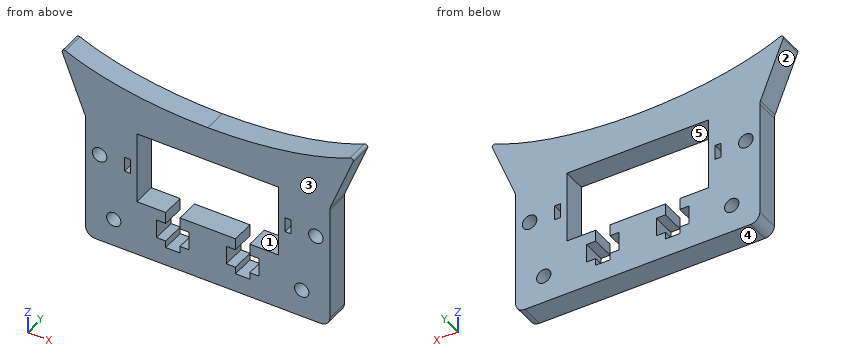
from build123d import *

# Parameters (mm, degrees)
SKETCH1_W           = 105
SKETCH1_H           = 70
BOSS_EXTRUDE1_DEPTH = 10
SKETCH2_W           = 61
SKETCH2_H           = 31
CUT_EXTRUDE1_DEPTH  = 11
SKETCH3_W           = 6.15
SKETCH3_H           = 5
SKETCH3_H_2         = 3
CUT_EXTRUDE2_DEPTH  = 10
SKETCH4_R           = 3.125
SKETCH4_W           = 2.5
SKETCH4_H           = 6.35
CUT_EXTRUDE3_DEPTH  = 11
BOSS_EXTRUDE2_DEPTH = 10
SKETCH6_R           = 3.075
CUT_EXTRUDE4_DEPTH  = 11.0000001
FILLET2_R           = 1
FILLET1_R           = 4


with BuildPart() as part:
    # Sketch1 → Boss-Extrude1 (new body)
    with BuildSketch(Plane(origin=(0, 0, 0), x_dir=(1, 0, 0), z_dir=(0, 1, 0))):
        Rectangle(SKETCH1_W, SKETCH1_H)
    extrude(amount=BOSS_EXTRUDE1_DEPTH)

    # Sketch2 → Cut-Extrude1 (cut, through all)
    with BuildSketch(Plane(origin=(0, 10, 0), x_dir=(1, 0, 0), z_dir=(0, 1, 0))):
        with Locations((0, -4.5)):
            Rectangle(SKETCH2_W, SKETCH2_H)
    extrude(amount=-CUT_EXTRUDE1_DEPTH, mode=Mode.SUBTRACT)

    # Sketch3 → Cut-Extrude2 (cut)
    with BuildSketch(Plane(origin=(0, 10, 0), x_dir=(1, 0, 0), z_dir=(0, 1, 0))):
        with Locations((-15, 13.5)):
            Rectangle(SKETCH3_W, SKETCH3_H)
        Polygon((-18.075, 24), (-22, 24), (-22, 16), (-18.075, 16), (-11.925, 16), (-8, 16), (-8, 24), (-11.925, 24), (-11.925, 21), (-18.075, 21), align=None)
        with Locations((-15, 22.5)):
            Rectangle(SKETCH3_W, SKETCH3_H_2)
        with Locations((-15, 25.5)):
            Rectangle(SKETCH3_W, SKETCH3_H_2)
    cut_extrude2 = extrude(amount=-CUT_EXTRUDE2_DEPTH, mode=Mode.SUBTRACT)

    # Sketch4 → Cut-Extrude3 (cut, through all)
    with BuildSketch(Plane(origin=(0, 10, 0), x_dir=(1, 0, 0), z_dir=(0, 1, 0))):
        with Locations((-46.5, -4)):
            Circle(SKETCH4_R)
        with Locations((-34.5, -4)):
            Rectangle(SKETCH4_W, SKETCH4_H)
    cut_extrude3 = extrude(amount=-CUT_EXTRUDE3_DEPTH, mode=Mode.SUBTRACT)

    # Sketch5 → Boss-Extrude2 (add)
    with BuildSketch(Plane(origin=(0, 0, 0), x_dir=(1, 0, 0), z_dir=(0, 1, 0))):
        with BuildLine():
            Line((0, -35), (-52.5, -19.039128985))
            Line((-52.5, -19.039128985), (-63.478993436, -46.742400328))
            add(Edge.make_bspline(
                [(0, -35), (-39.462588608, -35), (-63.478993436, -46.742400328)],
                knots=[4.71238898, 4.71238898, 4.71238898, 5.628907116, 5.628907116, 5.628907116], degree=2, weights=[1, 0.896824023, 1]))
        make_face()
    boss_extrude2 = extrude(amount=BOSS_EXTRUDE2_DEPTH)

    # Sketch6 → Cut-Extrude4 (cut, through all)
    with BuildSketch(Plane(origin=(0, 10, 0), x_dir=(1, 0, 0), z_dir=(0, 1, 0))):
        with Locations((-40.420875644, 23.095045258)):
            Circle(SKETCH6_R)
    cut_extrude4 = extrude(amount=-CUT_EXTRUDE4_DEPTH, mode=Mode.SUBTRACT)

    # Mirror1: Cut-Extrude2, Cut-Extrude3, Boss-Extrude2, Cut-Extrude4 across plane
    add(cut_extrude2.mirror(Plane(origin=(0, 0, 0), x_dir=(0, 0, 1), z_dir=(1, 0, 0))), mode=Mode.SUBTRACT)
    add(cut_extrude3.mirror(Plane(origin=(0, 0, 0), x_dir=(0, 0, 1), z_dir=(1, 0, 0))), mode=Mode.SUBTRACT)
    add(boss_extrude2.mirror(Plane(origin=(0, 0, 0), x_dir=(0, 0, 1), z_dir=(1, 0, 0))))
    add(cut_extrude4.mirror(Plane(origin=(0, 0, 0), x_dir=(0, 0, 1), z_dir=(1, 0, 0))), mode=Mode.SUBTRACT)

    # Fillet2
    fillet2_edges = [part.edges().sort_by_distance(p)[0] for p in [
        (-63.478993436, 5, 46.742400328),
        (63.478993436, 5, 46.742400328),
    ]]
    fillet(fillet2_edges, radius=FILLET2_R)

    # Fillet1
    fillet1_edges = [part.edges().sort_by_distance(p)[0] for p in [
        (52.5, 5, 19.039128985),
        (-52.5, 5, -35),
        (52.5, 5, -35),
        (-52.5, 5, 19.039128985),
    ]]
    fillet(fillet1_edges, radius=FILLET1_R)


solid = part.part
The listing builds one solid part. Answer for the finished solid, in the listing's coordinates (mm). Face numbers are marked on the shaded views. A direction names the side the tool comes from. Give positions to 0.01 mm unless a question says otherwise; leave off trailing zeros. Loops run counter-clockwise (first coordinate to the right, second up) from the corner with the lowest first, then second, coordinate; pieces in that order, holes last. Notation, with made-up numbers: M 13,68 L 46,68 A17 cw 46,93 Z; hole C -29,-26 d10. An arc over 180 degrees is marked long. Answer as CSV lines item,"result".
Item 1: The part is cut by section A-A (z = 4). Give the vertices of the cut face in (x, y) (3 decimals), and give its area (3 significant figures).
Values follow:
outline,"M -52.5,0 L -49.625,0 L -49.625,10 L -52.5,10 Z; M -43.375,0 L -35.75,0 L -35.75,10 L -43.375,10 Z; M -33.25,0 L -30.5,0 L -30.5,10 L -33.25,10 Z; M 30.5,0 L 33.25,0 L 33.25,10 L 30.5,10 Z; M 35.75,0 L 43.375,0 L 43.375,10 L 35.75,10 Z; M 49.625,0 L 52.5,0 L 52.5,10 L 49.625,10 Z"
area,"265 mm^2"
Item 2: Given pin 1 Ø3 at (y, z) = (7, -7.5) entering from -X; pin 2 Ø2 at (x, y) = (20.5, 4) entering from +Z; pin 3 Ø10 at (x, z) = (40.42, -23.1) entering from +Y; pin 4 Ø5 at (y, z) = (5.5, 31) entering from +X, each flat-ended and moving along its own axis, determine where each tip first touches the part or whether it passes through.
Values follow:
pin 1,"stops at x = -52.5"
pin 2,"stops at z = 36.1"
pin 3,"stops at y = 10"
pin 4,"stops at x = 58.23"
Item 3: Straight lines are drawn through the part: line 1 along X through (y, z) = (6.5, 4) (3 decimals); line 2 along Z through (x, y) = (-18, 3.25); line 3 along X through (y, z) = (8.75, -7). For each, find the intervals that lie inside material, in ascending order. Write a range as [from, to].
Values follow:
line 1,"x = [-52.5, -49.625], [-43.375, -35.75], [-33.25, -30.5], [30.5, 33.25], [35.75, 43.375], [49.625, 52.5]"
line 2,"z = [-35, -27], [20, 35.77]"
line 3,"x = [-52.5, -30.5], [30.5, 52.5]"
Item 4: The part is cut by section C-C (y = 4). Give the number of separate pieces and of enclosed holes in the cut face, and give its area (3 significant figures).
Values follow:
separate pieces,"1"
enclosed holes,"7"
area,"5,470 mm^2"
Item 5: The part is cut by section B-B (z = 14.5). Give the vertices of the cut face in (x, y).
Values follow:
outline,"M -52.5,0 L -30.5,0 L -30.5,10 L -52.5,10 Z; M 30.5,0 L 52.5,0 L 52.5,10 L 30.5,10 Z"
Item 6: Which of the six approach directions +Z, -Z, +X, -X, +Y, -Y give full straight-line access (tool end or side, diameter ignored) to the marked faces 4 and 5?
Values follow:
face 4,"-Z, +X, -X, +Y, -Y"
face 5,"+Y, -Y"
Item 7: The mould has two halves that part along Z. Classify the marked faces 1, 2 and 3: released by +Z, released by -Z, zero draft, split by the parting line, or undercut.
Values follow:
face 1,"undercut"
face 2,"released by -Z"
face 3,"zero draft"
